Autodesk Fusion 360 part; units mm, degrees
sketch "スケッチ1" plane through (0, 0, 0) normal (0, 1, 0) x (1, 0, 0)
  line L0 (-21, 0) -> (21, 0)
  line L1 (21, 0) -> (21, -72.5)
  line L2 (21, -72.5) -> (-21, -72.5)
  line L3 (-21, -72.5) -> (-21, 0)
  line L4 (6.5, -72.5) -> (-6.5, -72.5)
  line L5 (-6.5, -72.5) -> (-6.5, -96.5)
  line L6 (-6.5, -96.5) -> (6.5, -96.5)
  line L7 (6.5, -96.5) -> (6.5, -72.5)
  line L8 (-12.5, -160.5) -> (9, -160.5)
  line L9 (9, -160.5) -> (9, -96.5)
  line L10 (9, -96.5) -> (-12.5, -96.5)
  line L11 (-12.5, -96.5) -> (-12.5, -160.5)
  line L12 (-21, -67.5) -> (21, -67.5) construction
  circle A0 centre (-12, -67.5) radius 1.75
  circle A1 centre (12, -67.5) radius 1.75
  line L13 (0, -1.75) -> (0, -22.5)
  circle A2 centre (0, -155.5) radius 2
  dimension "d1" = 42
  dimension "d2" = 5
  dimension "d3" = 3.5
  dimension "d4" = 3.5
  dimension "d5" = 24
  dimension "d6" = 72.5
  dimension "d7" = 13
  dimension "d8" = 2.5
  dimension "d9" = 6
  dimension "d10" = 24
  dimension "d11" = 64
  dimension "d12" = 4
  dimension "d13" = 5
extrude "押し出し1" add sketch "スケッチ1" against normal blind 2 makes body 1
sketch "スケッチ2" plane through (0, 0, 0) normal (0, 1, 0) x (-1, 0, 0)
  circle A0 centre (12, 67.5) radius 1.75
  circle A1 centre (-12, 67.5) radius 1.75
  circle A2 centre (0, 155.5) radius 2
  line L0 (6.5, 72.5) -> (6.5, 96.5)
  line L1 (6.5, 96.5) -> (12.5, 96.5)
  line L2 (12.5, 96.5) -> (12.5, 160.5)
  line L3 (12.5, 160.5) -> (-9, 160.5)
  line L4 (-9, 160.5) -> (-9, 96.5)
  line L5 (-9, 96.5) -> (-6.5, 96.5)
  line L6 (-6.5, 96.5) -> (-6.5, 72.5)
  line L7 (-6.5, 72.5) -> (-21, 72.5)
  line L8 (-21, 72.5) -> (-21, 0)
  line L9 (-21, 0) -> (21, 0)
  line L10 (21, 0) -> (21, 72.5)
  line L11 (21, 72.5) -> (6.5, 72.5)
  line L12 (-21, 0) -> (-22.5, 0)
  line L13 (-22.5, 0) -> (-22.5, 74)
  line L14 (-22.5, 74) -> (-8, 74)
  line L15 (-8, 74) -> (-8, 95)
  line L16 (-8, 95) -> (-10.5, 95)
  line L17 (-10.5, 95) -> (-10.5, 160.5)
  line L18 (-10.5, 160.5) -> (-9, 160.5)
  line L19 (12.5, 160.5) -> (14, 160.5)
  line L20 (14, 160.5) -> (14, 95)
  line L21 (14, 95) -> (8, 95)
  line L22 (8, 95) -> (8, 74)
  line L23 (8, 74) -> (22.5, 74)
  line L24 (22.5, 74) -> (22.5, 0)
  line L25 (22.5, 0) -> (21, 0)
  dimension "d16" = 1.5
  dimension "d17" = 1.5
  dimension "d18" = 1.5
  dimension "d19" = 1.5
  dimension "d20" = 1.5
  dimension "d22" = 1.5
  dimension "d23" = 1.5
  dimension "d24" = 1.5
  dimension "d25" = 1.5
  dimension "d26" = 1.5
extrude "押し出し2" add sketch "スケッチ2" against normal blind 15 contours L0 L1 L2 L10 L11 L19 L20 L21 L22 L23 L24 L25 | L4 L5 L6 L7 L8 L12 L13 L14 L15 L16 L17 L18 bodies 1
sketch "スケッチ3" plane through (0, -2, 0) normal (0, -1, 0) x (1, 0, 0)
  circle A0 centre (-12, 67.5) radius 1.75
  circle A1 centre (12, 67.5) radius 1.75
  circle A2 centre (0, 155.5) radius 2
  line L0 (-6.5, 96.5) -> (-6.5, 72.5)
  line L1 (-6.5, 72.5) -> (-21, 72.5)
  line L2 (-21, 72.5) -> (-21, 0)
  line L3 (-21, 0) -> (21, 0)
  line L4 (21, 0) -> (21, 72.5)
  line L5 (21, 72.5) -> (6.5, 72.5)
  line L6 (6.5, 72.5) -> (6.5, 96.5)
  line L7 (6.5, 96.5) -> (9, 96.5)
  line L8 (9, 96.5) -> (9, 160.5)
  line L9 (9, 160.5) -> (-12.5, 160.5)
  line L10 (-12.5, 160.5) -> (-12.5, 96.5)
  line L11 (-12.5, 96.5) -> (-6.5, 96.5)
  line L12 (-21, 0) -> (21, 0)
  line L13 (21, 0) -> (21, 10)
  line L14 (21, 10) -> (-21, 10)
  line L15 (-21, 10) -> (-21, 0)
  line L16 (-21, 12.6) -> (21, 12.6)
  line L17 (21, 12.6) -> (21, 22.6)
  line L18 (21, 22.6) -> (-21, 22.6)
  line L19 (-21, 22.6) -> (-21, 12.6)
  dimension "d29" = 10
  dimension "d30" = 10
  dimension "d31" = 2.6
extrude "押し出し3" add sketch "スケッチ3" along normal up to surface (13 mm away) contours L2 L4 L16 L17 L18 L19 | L2 L3 L4 L12 L13 L14 L15 bodies 1
sketch "スケッチ4" plane through (0, 0, 0) normal (0, 0, -1) x (1, 0, 0)
  line L0 (-22.5, 0) -> (22.5, 0)
  line L1 (22.5, 0) -> (22.5, 15)
  line L2 (22.5, 15) -> (-22.5, 15)
  line L3 (-22.5, 15) -> (-22.5, 0)
  arc A0 (-12.5, 15) -> (12.5, 15) centre (0, 15) ccw
  dimension "d34" = 25
extrude "押し出し4" cut sketch "スケッチ4" against normal up to surface (22.6 mm away) contours L2 A0 bodies 1
sketch "スケッチ10" plane through (0, -2, 0) normal (0, -1, 0) x (1, 0, 0)
  circle A0 centre (12, 67.5) radius 1.75
  circle A1 centre (0, 155.5) radius 2
  circle A2 centre (-12, 67.5) radius 1.75
  line L0 (-21, 22.6) -> (21, 22.6)
  line L1 (21, 22.6) -> (21, 72.5)
  line L2 (21, 72.5) -> (6.5, 72.5)
  line L3 (6.5, 72.5) -> (6.5, 96.5)
  line L4 (6.5, 96.5) -> (9, 96.5)
  line L5 (9, 96.5) -> (9, 160.5)
  line L6 (9, 160.5) -> (-12.5, 160.5)
  line L7 (-12.5, 160.5) -> (-12.5, 96.5)
  line L8 (-12.5, 96.5) -> (-6.5, 96.5)
  line L9 (-6.5, 96.5) -> (-6.5, 72.5)
  line L10 (-6.5, 72.5) -> (-21, 72.5)
  line L11 (-21, 72.5) -> (-21, 22.6)
  circle A3 centre (0, 155.5) radius 4
  dimension "d48" = 8
extrude "押し出し9" add sketch "スケッチ10" along normal blind 6 contours A3 bodies 1
sketch "スケッチ9" plane through (0, -2, 0) normal (0, -1, 0) x (1, 0, 0)
  circle A0 centre (12, 67.5) radius 1.75
  circle A1 centre (-12, 67.5) radius 1.75
  line L0 (-21, 22.6) -> (21, 22.6)
  line L1 (21, 22.6) -> (21, 72.5)
  line L2 (21, 72.5) -> (6.5, 72.5)
  line L3 (6.5, 72.5) -> (6.5, 96.5)
  line L4 (6.5, 96.5) -> (9, 96.5)
  line L5 (9, 96.5) -> (9, 160.5)
  line L6 (9, 160.5) -> (-12.5, 160.5)
  line L7 (-12.5, 160.5) -> (-12.5, 96.5)
  line L8 (-12.5, 96.5) -> (-6.5, 96.5)
  line L9 (-6.5, 96.5) -> (-6.5, 72.5)
  line L10 (-6.5, 72.5) -> (-21, 72.5)
  line L11 (-21, 72.5) -> (-21, 22.6)
  line L12 (-21, 72.5) -> (21, 72.5)
  line L13 (21, 72.5) -> (21, 62.5)
  line L14 (21, 62.5) -> (-21, 62.5)
  line L15 (-21, 62.5) -> (-21, 72.5)
  circle A2 centre (0, 155.5) radius 4
  dimension "d45" = 10
extrude "押し出し8" add sketch "スケッチ9" along normal blind 1 contours L1 L2 L10 L11 L12 L13 L14 L15 bodies 1
ref_plane "作業平面1" through (0, -20, 80.25) normal (0, -1, 0) x (0, 0, -1)
sketch "スケッチ6" plane through (0, -20, 0) normal (0, -1, 0) x (-1, 0, 0)
  line L0 (-22.5, 0) -> (22.5, 0)
  line L1 (22.5, 0) -> (22.5, -22.6)
  line L2 (22.5, -22.6) -> (-22.5, -22.6)
  line L3 (-22.5, -22.6) -> (-22.5, 0)
  line L4 (-22.5, 0) -> (-22.5, -74)
  line L5 (-12.5, -22.6) -> (-21, -22.6)
  line L6 (-12.5, 0) -> (-22.5, 0)
  line L7 (22.5, -74) -> (22.5, 0)
extrude "押し出し5" add sketch "スケッチ6" along normal blind 15 separate body makes body 2
sketch "スケッチ7" plane through (0, 0, 0) normal (0, 0, -1) x (1, 0, 0)
  line L0 (-22.5, 20) -> (22.5, 20)
  line L1 (22.5, 20) -> (22.5, 35)
  line L2 (22.5, 35) -> (-22.5, 35)
  line L3 (-22.5, 35) -> (-22.5, 20)
  arc A0 (12.5, 20) -> (-12.5, 20) centre (0, 20) ccw
  dimension "d40" = 25
extrude "押し出し6" cut sketch "スケッチ7" against normal up to surface (22.6 mm away) contours L0 A0 bodies 2
sketch "スケッチ8" plane through (0, -20, 0) normal (0, 1, 0) x (-1, 0, 0)
  line L0 (-12.5, 0) -> (-12.5, 22.6)
  line L1 (-12.5, 22.6) -> (-22.5, 22.6)
  line L2 (-22.5, 22.6) -> (-22.5, 0)
  line L3 (-22.5, 0) -> (-12.5, 0)
  line L4 (21, 12.6) -> (-21, 12.6)
  line L5 (-21, 12.6) -> (-21, 10)
  line L6 (-21, 10) -> (21, 10)
  line L7 (21, 10) -> (21, 12.6)
  point P0 (21, 12.6)
  point P1 (21, 10)
  point P2 (-21, 12.6)
extrude "押し出し7" cut sketch "スケッチ8" against normal blind 13 contours L0 L4 L5 L6 | L0 L4 L6 L7 bodies 2
sketch "スケッチ11" plane through (0, -15, 0) normal (0, -1, 0) x (1, 0, 0)
  line L0 (-12.5, 0) -> (-12.5, 10)
  line L1 (-12.5, 10) -> (-21, 10)
  line L2 (-21, 10) -> (-21, 12.6)
  line L3 (-21, 12.6) -> (-12.5, 12.6)
  line L4 (-12.5, 12.6) -> (-12.5, 22.6)
  line L5 (-12.5, 22.6) -> (-21, 22.6)
  line L6 (-21, 22.6) -> (-21, 72.5)
  line L7 (-21, 72.5) -> (-6.5, 72.5)
  line L8 (-6.5, 72.5) -> (-6.5, 96.5)
  line L9 (-6.5, 96.5) -> (-12.5, 96.5)
  line L10 (-12.5, 96.5) -> (-12.5, 160.5)
  line L11 (-12.5, 160.5) -> (-14, 160.5)
  line L12 (-14, 160.5) -> (-14, 95)
  line L13 (-14, 95) -> (-8, 95)
  line L14 (-8, 95) -> (-8, 74)
  line L15 (-8, 74) -> (-22.5, 74)
  line L16 (-22.5, 74) -> (-22.5, 0)
  line L17 (-22.5, 0) -> (-12.5, 0)
  line L18 (-17.5, 17.6) -> (17.5, 17.6) construction
  line L19 (17.5, 17.6) -> (17.5, 5) construction
  line L20 (17.5, 5) -> (-17.5, 5) construction
  line L21 (-17.5, 5) -> (-17.5, 17.6) construction
  line L22 (22.5, 0) -> (22.5, 74)
  circle A0 centre (-17.5, 17.6) radius 2.5
  circle A1 centre (17.5, 17.6) radius 2.5
  circle A2 centre (-17.5, 5) radius 2.5
  circle A3 centre (17.5, 5) radius 2.5
  dimension "d51" = 5
  dimension "d52" = 5
  dimension "d53" = 5
  dimension "d54" = 5
  dimension "d55" = 5
  dimension "d56" = 5
  dimension "d57" = 5
  dimension "d58" = 5
extrude "押し出し10" cut sketch "スケッチ11" against normal blind 10 contours A0 | A1 | A2 | A3 bodies 1
sketch "スケッチ12" plane through (0, -20, 0) normal (0, 1, 0) x (-1, 0, 0)
  line L0 (12.5, 12.6) -> (21, 12.6)
  line L1 (21, 12.6) -> (21, 10)
  line L2 (21, 10) -> (12.5, 10)
  line L3 (12.5, 10) -> (12.5, 0)
  line L4 (12.5, 0) -> (22.5, 0)
  line L5 (22.5, 0) -> (22.5, 22.6)
  line L6 (22.5, 22.6) -> (12.5, 22.6)
  line L7 (12.5, 22.6) -> (12.5, 12.6)
  circle A0 centre (17.5, 17.6) radius 2.5
  circle A1 centre (17.5, 17.6) radius 2.5
  circle A2 centre (17.5, 5) radius 2.5
  circle A3 centre (-17.5, 17.6) radius 2.5
  circle A4 centre (-17.5, 5) radius 2.5
  circle A5 centre (-17.5, 17.6) radius 2.25
  circle A6 centre (-17.5, 5) radius 2.25
  circle A7 centre (17.5, 17.6) radius 2.25
  circle A8 centre (17.5, 5) radius 2.25
  dimension "d63" = 4.5
  dimension "d64" = 4.5
  dimension "d65" = 4.5
  dimension "d66" = 4.5
extrude "押し出し12" add sketch "スケッチ12" along normal blind 6 contours A5 | A6 | A7 | A8 bodies 2
sketch "スケッチ14" plane through (0, 0, 0) normal (0, 1, 0) x (-1, 0, 0)
  circle A0 centre (0, 155.5) radius 2
  circle A1 centre (12, 67.5) radius 1.75
  circle A2 centre (-12, 67.5) radius 1.75
  line L0 (14, 160.5) -> (-10.5, 160.5)
  line L1 (-10.5, 160.5) -> (-10.5, 95)
  line L2 (-10.5, 95) -> (-8, 95)
  line L3 (-8, 95) -> (-8, 74)
  line L4 (-8, 74) -> (-22.5, 74)
  line L5 (-22.5, 74) -> (-22.5, 0)
  line L6 (-22.5, 0) -> (22.5, 0)
  line L7 (22.5, 0) -> (22.5, 74)
  line L8 (22.5, 74) -> (8, 74)
  line L9 (8, 74) -> (8, 95)
  line L10 (8, 95) -> (14, 95)
  line L11 (14, 95) -> (14, 160.5)
  line L12 (14, 149) -> (15.5, 149)
  line L13 (15.5, 149) -> (14, 150.5)
  line L14 (14, 126.5) -> (15.5, 126.5)
  line L15 (15.5, 126.5) -> (14, 125)
  line L16 (-10.5, 150.5) -> (-12, 149)
  line L17 (-12, 149) -> (-10.5, 149)
  line L18 (-10.5, 126.5) -> (-12, 126.5)
  line L19 (-12, 126.5) -> (-10.5, 125)
  dimension "d79" = 10
  dimension "d80" = 10
  dimension "d81" = 1.5
  dimension "d82" = 1.5
  dimension "d83" = 22.5
  dimension "d84" = 1.5
  dimension "d85" = 1.5
  dimension "d86" = 1.5
  dimension "d88" = 1.5
  dimension "d89" = 1.5
extrude "押し出し13" add sketch "スケッチ14" against normal up to surface (15 mm away) contours L11 L12 L13 | L1 L16 L17 | L11 L14 L15 | L1 L18 L19 bodies 1
hidden bodies 2
CAD build for the part. Positions are in the model's coordinates, mm. A direction names the side the tool comes from. Give positions to 0.01 mm unless a question says otherwise; leave off trailing zeros. Order: outer loops, then holes, each group sorted by start corner. A loop starts at its lowest first (then second) coordinate and runs counter-clockwise, first axis right, second up. Notation, with made-up numbers: M 8.5,57 L 64.5,57 A33 cw 64.5,91 Z; hole C 58.5,-9.5 d5. An arc over 180 degrees is marked long. Put each result on its own line as item: value. Start each with the question number.
(1) Mould opens along X. For faces 6 (the flat face through (10.5, -7, 138)), 7 (the cylindrical face through (15, -10.1, 17.7)), 8 (the flat face through (-14, -7, 138)) say: +X half, -X half, draft (parallel to the pull), parting line (faces both ways), or undercut.
(2) Flat gauge pins, fed straight in: pin 1 Ø3.5 at (x, z) = (0, 155.5) entering from -Y; pin 2 Ø2 at (x, y) = (-4, -7.5) entering from +Z; pin 3 Ø4 at (y, z) = (-10.5, 80) entering from +X; pin 4 Ø4 at (y, z) = (-6, 127) entering from -X. Where does each tip first touch, or does it go through?
(3) Saw through at C-C, the plane z = 67.5. Write the cut outline in (x, y), then the cut area to 3 significant figures.
(4) Drill centre lines: line 1 along X through (y, z) = (-0.65, 67.5); line 2 along Z through (x, y) = (-17.5, -8.5); line 3 along Z through (x, y) = (13.5, -10.5). Where is each one in solid material? Low to high.
(5) Saw through at B-B, the plane x = 0. Write the cut outline in (y, z).
(6) Which spindle directions (+Z, -Z, +X, -X, +Y, -Y) get a long thin tool onto all of the face, cutting with end or side? Do faces 1 (the flat face through (14, -9, 72.5)), 2 (the flat face through (-8, -7, 85)), 3 (the flat face through (15, -7, 74)), 4 (the flat face through (10.5, -7, 155)), 5 (the flat face through (-6.5, -8, 84)). Say none if no direction does.
(7) Saw through at A-A, the plane z = 155.5. Write the cut outline in (x, y), then the cut area to 3 significant figures.
(8) Saw through at D-D, the plane z = 132.5. Write the cut outline in (x, y), then the cut area to 3 significant figures.
Check result:
1. face 6: +X half
1. face 7: undercut
1. face 8: -X half
2. pin 1: passes through
2. pin 2: stops at z = 158.15
2. pin 3: stops at x = 8
2. pin 4: stops at x = -15.5
3. outline: M -22.5,-15 L -21,-15 L -21,-3 L -13.75,-3 L -13.75,0 L -22.5,0 Z; M -10.25,-3 L 10.25,-3 L 10.25,0 L -10.25,0 Z; M 13.75,-3 L 21,-3 L 21,-15 L 22.5,-15 L 22.5,0 L 13.75,0 Z
3. area: 150 mm2
4. line 1: x = -22.5 to -13.75, -10.25 to 10.25, 13.75 to 22.5
4. line 2: z = 0 to 2.5, 7.5 to 10, 12.6 to 15.1, 20.1 to 22.6, 72.5 to 74
4. line 3: z = 0 to 10, 12.6 to 22.6, 72.5 to 74
5. outline: M -8,151.5 L -2,151.5 L -2,72.5 L -3,72.5 L -3,62.5 L -2,62.5 L -2,22.6 L -2.5,22.6 L -2.5,12.6 L -2,12.6 L -2,10 L -2.5,10 L -2.5,0 L 0,0 L 0,153.5 L -8,153.5 Z; M -8,157.5 L 0,157.5 L 0,160.5 L -2,160.5 L -2,159.5 L -8,159.5 Z
6. face 1: -Y
6. face 2: -X, +Y, -Y
6. face 3: +X, +Y, -Y
6. face 4: +Z, +X, +Y, -Y
6. face 5: +Z, -Y
7. outline: M -14,-15 L -12.5,-15 L -12.5,-2 L -4,-2 L -4,-8 L -2,-8 L -2,0 L -14,0 Z; M 2,-8 L 4,-8 L 4,-2 L 9,-2 L 9,-15 L 10.5,-15 L 10.5,0 L 2,0 Z
7. area: 104 mm2
8. outline: M -14,-15 L -12.5,-15 L -12.5,-2 L 9,-2 L 9,-15 L 10.5,-15 L 10.5,0 L -14,0 Z
8. area: 88.0 mm2
